Build history of the part. All positions in model axes, mm. A direction names the side the tool comes from. Give positions to 0.01 mm unless a question says otherwise; leave off trailing zeros. Loops run counter-clockwise (first coordinate to the right, second up) from the corner with the lowest first, then second, coordinate; pieces in that order, holes last.
1) Band-saw the part on C-C on z = 0. List the corners of the cut face in (x, y).
2) Flat gauge pins, fed straight in: P1, Ø4, axis at x = 16, y = 1, coming from the -Z side; P2, Ø4, axis at x = -22.5, y = 4, coming from the +Z side; P3, Ø5.5, axis at x = -20.75, z = 35.94, coming from the +Y side; P4, Ø2.5, axis at x = 20.75, z = -35.94, coming from the +Y side. Where does each tip first touch, or does it go through?
3) Wall check: line 1 (Z direction, x = 20.75, y = 6.25); line 2 (X direction, y = 2.75, z = 20); line 3 (Y direction, x = 25.5, z = -38). Give the ranges that are in metal, low to high.
4) Two-plate mould, pull along Z, no slides. Class faces 3 (the flat face through (-33, 0, -20)), 4 (the cylindrical face through (-17.235, 3.944, 41.569)), 5 (the cylindrical face through (-23.122, 4.437, -30.156)): +Z half, -Z half, draft (parallel to the pull), parting line (faces both ways), or undercut.
5) Band-saw the part on A-A on x = 0. List the corners of the cut face in (y, z), then the cut area to 3 significant figures.
6) Band-saw the part on B-B on z = -28.5. List the corners of the cut face in (x, y).
7) Band-saw the part on D-D on x = 20.75. List the corners of the cut face in (y, z), then the cut area to 3 significant figures.
8) 3-axis set-ups, long thin cutter, end or side, ignore diameter. For faces 1 (the flat face through (38.1, 8, -24.3)), 2 (the cylindrical face through (46.1, 8.5, -6.1)): which of +Z, -Z, +X, -X, +Y, -Y reach the whole face in a straight line?
```python
from build123d import *

# Parameters (mm, degrees)
SKETCH_2_R         = 45
SKETCH_2_R_2       = 38
EXTRUDE_1_DEPTH    = 8
SKETCH_6_R         = 46.5
SKETCH_6_R_2       = 38
EXTRUDE_3_DEPTH    = 1
HOLE_WIZARD_M4_1_D = 3.3


with BuildPart() as part:
    # 草图2 → 凸台-拉伸1 (new body)
    with BuildSketch(Plane(origin=(0, 0, 0), x_dir=(1, 0, 0), z_dir=(0, 1, 0))):
        with Locations(Location((0, 0, 0), (0, 0, 270))):
            Circle(SKETCH_2_R)
        with Locations(Location((0, 0, 0), (0, 0, 270))):
            Circle(SKETCH_2_R_2, mode=Mode.SUBTRACT)
    extrude(amount=EXTRUDE_1_DEPTH)

    # 草图6 → 凸台-拉伸3 (add)
    with BuildSketch(Plane(origin=(0, 8, 0), x_dir=(1, 0, 0), z_dir=(0, 1, 0))):
        with Locations(Location((0, 0, 0), (0, 0, 270))):
            Circle(SKETCH_6_R)
        with Locations(Location((0, 0, 0), (0, 0, 270))):
            Circle(SKETCH_6_R_2, mode=Mode.SUBTRACT)
    extrude(amount=EXTRUDE_3_DEPTH)

    # M4 螺纹孔1 (through all)
    with Locations(Plane(origin=(0, 9, 0), x_dir=(1, 0, 0), z_dir=(0, 1, 0))):
        with Locations((-20.75, 35.940054257), (20.75, 35.940054257), (41.5, 0), (20.75, -35.940054257), (-20.75, -35.940054257), (-41.5, 0)):
            Hole(HOLE_WIZARD_M4_1_D / 2)


solid = part.part
```
Findings below:
1. outline: (-46.5, 8) - (-45, 8) - (-45, 0) - (-43.15, 0) - (-43.15, 9) - (-46.5, 9) - close; (-39.85, 0) - (-38, 0) - (-38, 9) - (-39.85, 9) - close; (38, 0) - (39.85, 0) - (39.85, 9) - (38, 9) - close; (43.15, 0) - (45, 0) - (45, 8) - (46.5, 8) - (46.5, 9) - (43.15, 9) - close
2. P1: stops at z = -42.77
2. P2: stops at z = 40.06
2. P3: stops at y = 9
2. P4: passes through
3. line 1: z = -39.93 to -37.59, -34.29 to -31.83, 31.83 to 34.29, 37.59 to 39.93
3. line 2: x = -40.31 to -32.31, 32.31 to 40.31
3. line 3: y = 8 to 9
4. face 3: draft
4. face 4: parting line
4. face 5: undercut
5. outline: (0, -45) - (8, -45) - (8, -46.5) - (9, -46.5) - (9, -38) - (0, -38) - close; (0, 38) - (9, 38) - (9, 46.5) - (8, 46.5) - (8, 45) - (0, 45) - close
5. area: 129 mm2
6. outline: (-36.74, 8) - (-34.82, 8) - (-34.82, 0) - (-25.13, 0) - (-25.13, 9) - (-36.74, 9) - close; (25.13, 0) - (34.82, 0) - (34.82, 8) - (36.74, 8) - (36.74, 9) - (25.13, 9) - close
7. outline: (0, -39.93) - (8, -39.93) - (8, -41.61) - (9, -41.61) - (9, -37.59) - (0, -37.59) - close; (0, -34.29) - (9, -34.29) - (9, -31.83) - (0, -31.83) - close; (0, 31.83) - (9, 31.83) - (9, 34.29) - (0, 34.29) - close; (0, 37.59) - (9, 37.59) - (9, 41.61) - (8, 41.61) - (8, 39.93) - (0, 39.93) - close
7. area: 89.7 mm2
8. face 1: -Y
8. face 2: +Y, -Y
